Source: CAD feature listing. Evaluate the final solid. Frame: model axes, mm. Face numbers are marked on the shaded views. A direction names the side the tool comes from. Coordinates: 2 decimals unless noted, no trailing zeros. Loops run counter-clockwise (first coordinate to the right, second up) from the corner with the lowest first, then second, coordinate; pieces in that order, holes last.
Item 1: Line query: probe 1 along Y at (x, z) = (-57.15, 21); probe 2 along Z at (x, y) = (-21.5, -5); probe 3 along Y at (x, z) = (-21, 4). Output: solid intervals per line, ascending.
Item 2: Reachability of the marked faces 4 and 5 from +Z, -Z, +X, -X, +Y, -Y: full face, straight path, thin tool, end or side. Return the list, or none.
Item 3: Pull-direction query (X, two-part tool) for the marked faces 1, 2 and 3; classes: +X half, -X half, draft (parallel to the pull), parting line (faces both ways), or undercut.
Item 4: Pin query (flat end, axial travel): pin 1 Ø12 at (x, z) = (-26.5, 21.5) entering from +Y; pin 2 Ø3 at (y, z) = (-19, 15.5) entering from +X; pin 3 Ø6 at (y, z) = (-10, 22.5) entering from +X; pin 4 Ø1.5 at (y, z) = (-21, 31.5) entering from +X. Return the tip coordinate at first contact, or that it passes through.
Item 5: Section query D-D, the plane x = -48.5. Return the cut outline in (y, z), then the cut area to 3 significant figures.
Item 6: Section query B-B, the plane x = -21. Return the cut outline in (y, z), then the cut area to 3 significant figures.
Item 7: Section query A-A, the plane z = 3. Return the cut outline in (x, y).
Item 8: Section query C-C, the plane z = 28.5. Return the cut outline in (x, y), then the cut area to 3 significant figures.
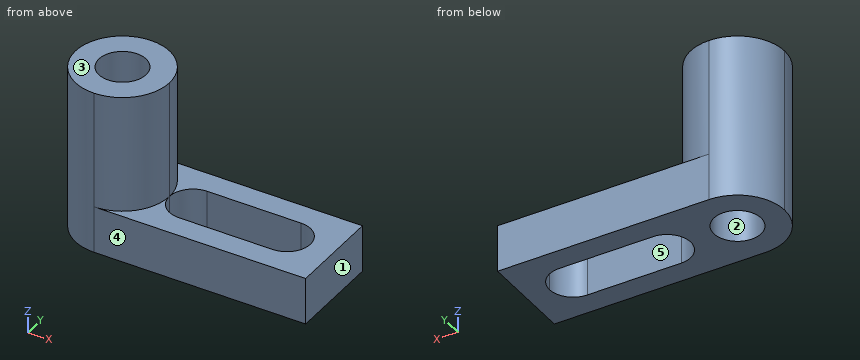
```python
from build123d import *

# Parameters (mm, degrees)
F0_W      = 69.85
F0_H      = 44.45
F1_DEPTH  = 25.4
F2_W      = 44.45
F2_H      = 31.75
F3_DEPTH  = 25.401
F5_DEPTH  = 44.451
F7_DEPTH  = 31.75
F9_DEPTH  = 44.451
F10_R     = 6.3621373658
F11_DEPTH = 44.451


with BuildPart() as f1:
    # F0 (on Front) → F1 (new body)
    with BuildSketch(Plane.XZ):
        with Locations((-34.925, 22.225)):
            Rectangle(F0_W, F0_H)
    extrude(amount=F1_DEPTH)

    # F2 (on face) → F3 (cut, through all)
    with BuildSketch(Plane.XZ.offset(25.4)):
        with Locations((-22.225, 28.575)):
            Rectangle(F2_W, F2_H)
    extrude(amount=-F3_DEPTH, mode=Mode.SUBTRACT)

    # F4 (on face) → F5 (cut, through all)
    with BuildSketch(Plane.XY.offset(44.45)):
        with BuildLine():
            ThreePointArc((-69.85, -12.7), (-66.1302561211, -3.7197438789), (-57.15, 0))
            Line((-57.15, 0), (-69.85, 0))
            Line((-69.85, 0), (-69.85, -12.7))
        make_face()
        with BuildLine():
            Line((-69.85, -25.4), (-57.15, -25.4))
            ThreePointArc((-57.15, -25.4), (-66.1302561211, -21.6802561211), (-69.85, -12.7))
            Line((-69.85, -12.7), (-69.85, -25.4))
        make_face()
    extrude(amount=-F5_DEPTH, mode=Mode.SUBTRACT)

    # F6 (on face) → F7 (cut)
    with BuildSketch(Plane.XY.offset(44.45)):
        with BuildLine():
            ThreePointArc((-57.15, 0), (-48.1697438789, -3.7197438789), (-44.45, -12.7))
            Line((-44.45, -12.7), (-44.45, 0))
            Line((-44.45, 0), (-57.15, 0))
        make_face()
        with BuildLine():
            Line((-44.45, -25.4), (-44.45, -12.7))
            ThreePointArc((-44.45, -12.7), (-48.1697438789, -21.6802561211), (-57.15, -25.4))
            Line((-57.15, -25.4), (-44.45, -25.4))
        make_face()
    extrude(amount=-F7_DEPTH, mode=Mode.SUBTRACT)

    # F8 (on face) → F9 (cut, through all)
    with BuildSketch(Plane(origin=(0, 0, 0), x_dir=(1, 0, 0), z_dir=(0, 0, -1))):
        with BuildLine():
            Line((-38.1, 6.3958125417), (-12.7, 6.3958125417))
            ThreePointArc((-12.7, 6.3958125417), (-8.2098719395, 8.2556844811), (-6.35, 12.7458125417))
            ThreePointArc((-6.35, 12.7458125417), (-8.2098719395, 17.2359406022), (-12.7, 19.0958125417))
            Line((-12.7, 19.0958125417), (-38.1, 19.0958125417))
            ThreePointArc((-38.1, 19.0958125417), (-42.5901280605, 17.2359406022), (-44.45, 12.7458125417))
            ThreePointArc((-44.45, 12.7458125417), (-42.5901280605, 8.2556844811), (-38.1, 6.3958125417))
        make_face()
    extrude(amount=-F9_DEPTH, mode=Mode.SUBTRACT)

    # F10 (on face) → F11 (cut, through all)
    with BuildSketch(Plane.XY.offset(44.45)):
        with Locations((-57.15, -12.7)):
            Circle(F10_R)
    extrude(amount=-F11_DEPTH, mode=Mode.SUBTRACT)


solid = f1.part
```
Verdict:
1. probe 1: y = -25.4 to -19.06, -6.34 to 0
1. probe 2: z = 0 to 12.7
1. probe 3: y = -25.4 to -19.1, -6.4 to 0
2. face 4: +Z, -Z, +X, -X, -Y
2. face 5: +Z, -Z
3. face 1: +X half
3. face 2: undercut
3. face 3: draft
4. pin 1: passes through
4. pin 2: stops at x = -45.39
4. pin 3: stops at x = -44.45
4. pin 4: stops at x = -46.94
5. outline: (-25.4, 0) - (0, 0) - (0, 12.7) - (-3.4, 12.7) - (-3.4, 44.45) - (-22, 44.45) - (-22, 12.7) - (-25.4, 12.7) - close
5. area: 913 mm2
6. outline: (-25.4, 0) - (-19.1, 0) - (-19.1, 12.7) - (-25.4, 12.7) - close; (-6.4, 0) - (0, 0) - (0, 12.7) - (-6.4, 12.7) - close
6. area: 161 mm2
7. outline: (-57.15, -25.4) - (0, -25.4) - (0, 0) - (-57.15, 0) arc R12.7 ccw to start; hole circle Ø12.72 at (-57.15, -12.7); hole (-38.1, -19.1) - (-12.7, -19.1) arc R6.35 ccw to (-12.7, -6.4) - (-38.1, -6.4) arc R6.35 ccw to start
8. outline: circle Ø25.4 at (-57.15, -12.7); hole circle Ø12.72 at (-57.15, -12.7)
8. area: 380 mm2
